Autodesk Inventor part; units mm, degrees
ref_plane "Plano de trabajo2" through (0, 0, 120) normal (0, 0, -1) x (-1, 0, 0)
ref_plane "YZ Plane" through (0, 0, 0) normal (1, 0, 0) x (0, 1, 0)
ref_plane "XZ Plane" through (0, 0, 0) normal (0, 1, 0) x (-1, 0, 0)
sketch "Boceto1" plane through (0, 0, 0) normal (0, 1, 0) x (-1, 0, 0)
  arc A0 (-25, 25) -> (25, 25) centre (0, 25) ccw
  arc A1 (45, 75) -> (-45, 75) centre (0, 75) ccw
  line L0 (25, 25) -> (25, 75)
  line L1 (-25, 25) -> (-25, 75)
  line L2 (45, 75) -> (25, 75)
  line L3 (-25, 75) -> (-45, 75)
  point P0 (0, 0)
  dimension "d3" = 50
  dimension "d4" = 90
extrude "Extrusión1" add sketch "Boceto1" along normal blind 18
ref_plane "Plano de trabajo2" through (0, 0, 120) normal (0, 0, -1) x (-1, 0, 0)
sketch "Boceto3" plane through (0, 0, 120) normal (0, 0, -1) x (-1, 0, 0)
  circle A0 centre (0, 9) radius 2
  line L0 (45, 18) -> (-45, 18)
  point P0 (0, 0)
  dimension "d13" = 4
  dimension "d14" = 9
extrude "Extrusión3" add sketch "Boceto3" against normal blind 2
sketch "Boceto4" plane through (0, 9, 122) normal (0, 0, 1) x (1, 0, 0)
  circle A0 centre (0, 0) radius 2
  point P0 (0, -9)
  dimension "d17" = 4
extrude "Extrusión4" cut sketch "Boceto4" against normal blind 157.75
properties part number "APM_001-1"
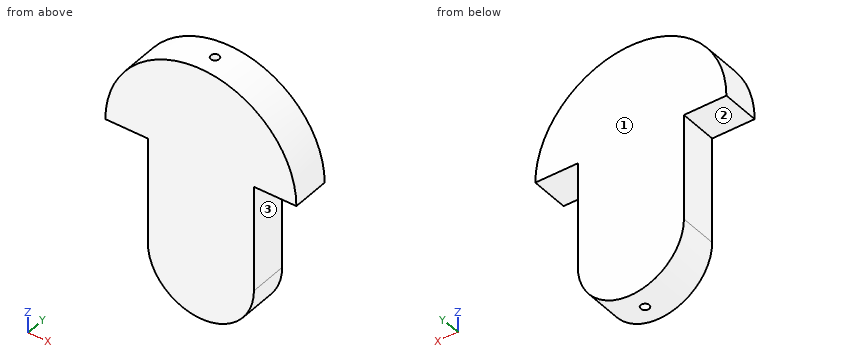
The listing builds one solid part. Answer for the finished solid, in the listing's coordinates (mm). Face numbers are marked on the shaded views. A direction names the side the tool comes from. Round coordinates to 2 decimals unless told otherwise and drop trailing zeros. Loops run counter-clockwise (first coordinate to the right, second up) from the corner with the lowest first, then second, coordinate; pieces in that order, holes last. Notation, with made-up numbers: (26, 69.5) - (59, 69.5) arc R30 cw to (59, 100.5) - close; hole circle Ø4 at (84, -19.5). An arc over 180 degrees is marked (long way). Use one line per item in the form item = value. Start each with the question number.
1. The part is cut by section A-A on x = 0. Determine the outline of the cut face in (y, z), then the cut area to 3 significant figures.
2. Given pin 1 Ø3 at (x, y) = (-3, 14.5) entering from -Z; pin 2 Ø3.5 at (x, y) = (0, 9) entering from -Z; pin 3 Ø6 at (y, z) = (8.5, 82) entering from +X; pin 4 Ø5.5 at (y, z) = (9, 43) entering from +X, each flat-ended and moving along its own axis, determine where each tip first touches the part or whether it passes through.
3. The part is cut by section B-B on y = 13.75. Determine the outline of the cut face in (x, z).
4. Consider line 1 (X direction, y = 9, z = 61.5); line 2 (Y direction, x = 0, z = 43.5); line 3 (X direction, y = 6, z = 52). Determine where each line is inside the solid, lowest interval first. Write a range as [from, to].
5. The part is cut by section D-D on x = 16. Determine the outline of the cut face in (y, z), then the cut area to 3 significant figures.
6. The part is cut by section C-C on z = 12.5. Determine the outline of the cut face in (x, y), then the cut area to 3 significant figures.
7. A tool of negligible diameter and unlimited length cuts with its end or side. For the marked faces 1, 2 and 3, from which of +Z, -Z, +X, -X, +Y, -Y can it reach the whole face along a straight path? Write none if from no direction.
Geometry check:
q1.outline = (0, 0) - (7, 0) - (7, 120) - (0, 120) - close; (11, 0) - (18, 0) - (18, 120) - (11, 120) - close
q1.area = 1,680 mm^2
q2.pin_1 = 0.05
q2.pin_2 = through
q2.pin_3 = 44.82
q2.pin_4 = 25
q3.outline = (-45, 75) - (-25, 75) - (-25, 25) arc R25 ccw to (25, 25) - (25, 75) - (45, 75) arc R45 ccw to start
q4.line_1 = [-25, -2], [2, 25]
q4.line_2 = [0, 7], [11, 18]
q4.line_3 = [-25, 25]
q5.outline = (0, 5.79) - (18, 5.79) - (18, 117.06) - (0, 117.06) - close
q5.area = 2,000 mm^2
q6.outline = (-21.65, 0) - (21.65, 0) - (21.65, 18) - (-21.65, 18) - close; hole circle Ø4 at (0, 9)
q6.area = 767 mm^2
q7.face_1 = +Z, -Z, +X, -X, +Y
q7.face_2 = -Z, -X, +Y, -Y
q7.face_3 = -Z, +X, +Y, -Y
